from build123d import *

# Parameters (mm, degrees)
SKETCH2_R           = 4
BOSS_EXTRUDE1_DEPTH = 81
CUT_EXTRUDE1_START  = 2
SKETCH3_W           = 2.5
SKETCH3_H           = 8
CUT_EXTRUDE1_DEPTH  = 10


with BuildPart() as part:
    # Sketch2 → Boss-Extrude1 (new, symmetric)
    with BuildSketch(Plane(origin=(0, 0, 0), x_dir=(0, 0, -1), z_dir=(1, 0, 0))):
        Circle(SKETCH2_R)
    extrude(amount=BOSS_EXTRUDE1_DEPTH, both=True)

    # Sketch3 → Cut-Extrude1 (cut)
    with BuildSketch(Plane(origin=(0, 0, 0), x_dir=(1, 0, 0), z_dir=(0, 1, 0)).offset(CUT_EXTRUDE1_START)):
        with Locations((-63, 0)):
            Rectangle(SKETCH3_W, SKETCH3_H)
        with Locations((-45, 0)):
            Rectangle(SKETCH3_W, SKETCH3_H)
        with Locations((-27, 0)):
            Rectangle(SKETCH3_W, SKETCH3_H)
        with Locations((-9, 0)):
            Rectangle(SKETCH3_W, SKETCH3_H)
        with Locations((9, 0)):
            Rectangle(SKETCH3_W, SKETCH3_H)
        with Locations((27, 0)):
            Rectangle(SKETCH3_W, SKETCH3_H)
        with Locations((45, 0)):
            Rectangle(SKETCH3_W, SKETCH3_H)
        with Locations((63, 0)):
            Rectangle(SKETCH3_W, SKETCH3_H)
    extrude(amount=CUT_EXTRUDE1_DEPTH, mode=Mode.SUBTRACT)


solid = part.part
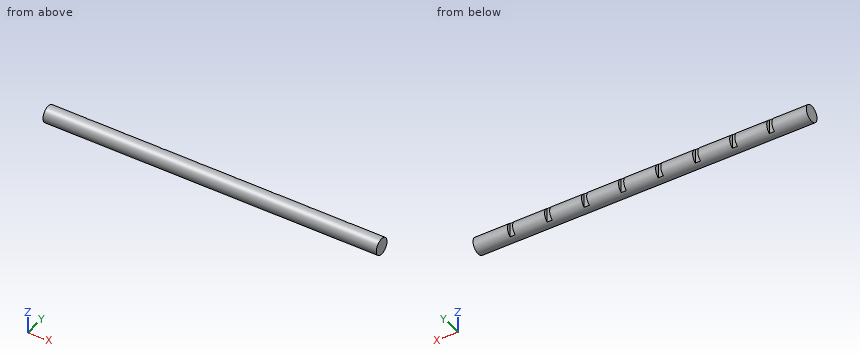
For this review, take the finished solid that the model builds, in its own axes (mm). Round coordinates to 2 decimals unless told otherwise and drop trailing zeros. Order: outer loops, then holes, each group sorted by start corner. A loop starts at its lowest first (then second) coordinate and runs counter-clockwise, first axis right, second up. Notation, with made-up numbers: (30, -1.5) -> (81, -1.5) arc R15 cw to (81, 22.5) -> close; hole circle Ø3 at (-7, 83). An arc over 180 degrees is marked (long way). Write item = value, one per line. Start each with the question number.
1) Take a section at A-A on x = 2. State the section outline as (y, z) points, plus the area to 3 significant figures.
2) Insertion check: pin 1 (0.8 mm diameter, centred on x = -45.5, z = 1.5, fed in from +Y); pin 2 (1.5 mm diameter, centred on x = -7, y = 3, fed in from -Z); pin 3 (2 mm diameter, centred on x = 7, z = -2.5, fed in from -Y). Each pin has a flat end and moves straight along its axis. Give the tip position at first contact, or say it passes through.
3) To check wall thickness, follow line 1 (Y direction, x = -46, z = -0.5); line 2 (Z direction, x = 66, y = 0.25); line 3 (Z direction, x = 72.5, y = 2). State the ranges of each line that lie inside material, in increasing order. Write a range as from..to.
Verdict:
q1.outline = circle Ø8 at (0, 0)
q1.area = 50.3 mm2
q2.pin_1 = 2
q2.pin_2 = -3.31
q2.pin_3 = -3.71
q3.line_1 = -3.97..2
q3.line_2 = -3.99..3.99
q3.line_3 = -3.46..3.46
